Source: three-view drawing plus pictorial views. Frame: mm from the lowest corner of the part. A direction names the side the tool comes from. Coordinates: 2 decimals unless noted, no trailing zeros. One line per question, with ' | ' between items.
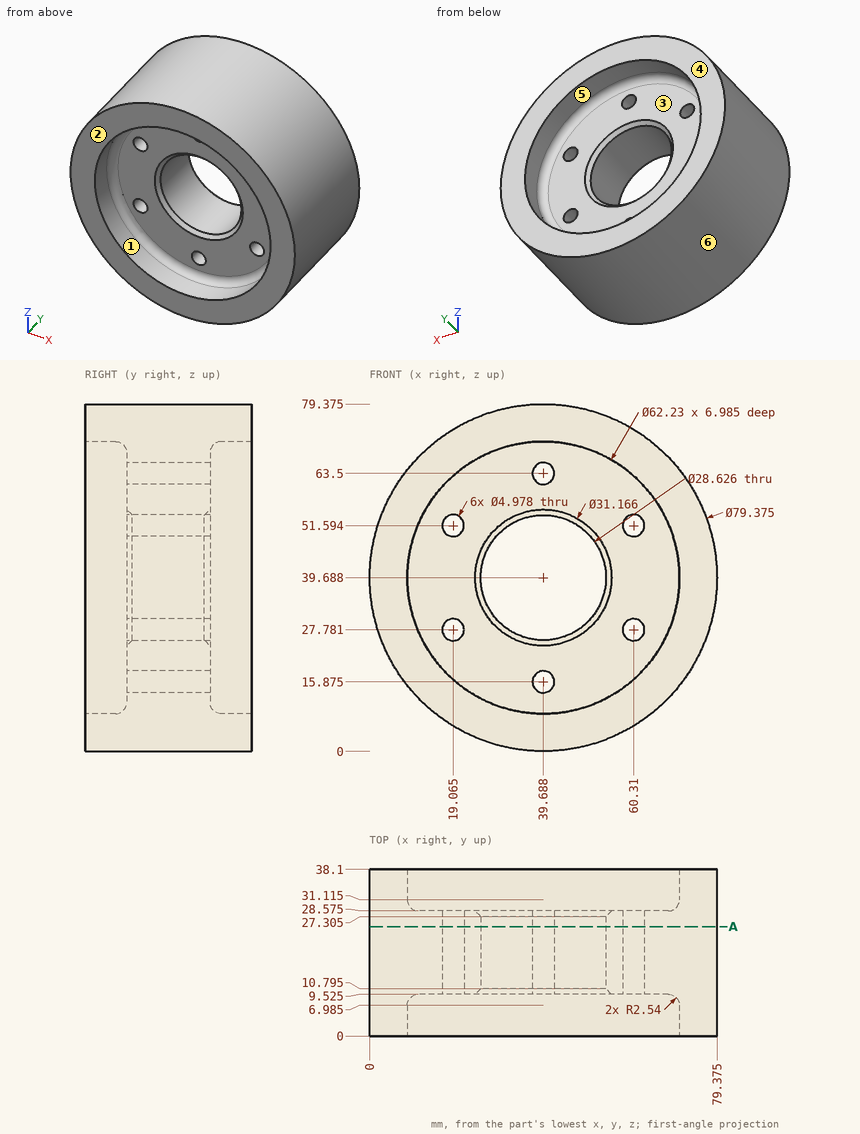
1. Material intervals for line 1 (Y direction, x = 22, z = 53.5) (1 decimal); line 2 (Z direction, x = 20.5, y = 22.5) (1 decimal); line 3 (Z direction, x = 46, y = 16) (1 decimal), sorted ascending. Write a range as [from, to].
Response values:
line 1: y = [9.5, 28.6] | line 2: z = [4.9, 25.7], [29.8, 49.6], [53.6, 74.4] | line 3: z = [0.5, 26.8], [52.5, 78.9]
2. Section A-A, the plane y = 25. Give the number of separate pieces and of enclosed holes in the cut face, and give its area (3 significant figures).
Response values:
separate pieces: 1 | enclosed holes: 7 | area: 4,190 mm^2
3. Draft query along X for the marked faces 3, 4, 5 and 6. Return one class per face: pulls with the +X half, pulls with the -X half, needs draft (parallel to the pull), parting line crosses it, or undercut.
Response values:
face 3: undercut | face 4: needs draft | face 5: undercut | face 6: parting line crosses it
4. Pin query (flat end, axial travel): P1, Ø4, axis at y = 17, z = 9, coming from the -X side; P2, Ø2, axis at y = 13.5, z = 57.5, coming from the -X side; P3, Ø3, axis at x = 65, z = 44.5, coming from the -Y side (1 decimal); P4, Ø4, axis at x = 39.69, z = 63.5, coming from the +Y side. Return the tip coordinate at first contact, or that it passes through.
Response values:
P1: stops at x = 12.26 | P2: stops at x = 3.74 | P3: stops at y = 9.5 | P4: passes through
5. Access query for the marked faces 1 and 2. Directions: +Z, -Z, +X, -X, +Y, -Y. A direction counts if a zero-diameter tool reaches every point of the face in a straight line with its end or side. Return the directions, or none.
Response values:
face 1: -Y | face 2: +Z, -Z, +X, -X, -Y
